Could you check a few things on this model? Use its own coordinates, in mm. A direction names the side the tool comes from. Round coordinates to 2 decimals unless told otherwise and drop trailing zeros. Loops run counter-clockwise (first coordinate to the right, second up) from the corner with the lowest first, then second, coordinate; pieces in that order, holes last. Notation, with made-up numbers: M 3.5,46 L 33.5,46 A19 cw 33.5,79 Z; hole C 22,44.5 d1. An arc over 180 degrees is marked long. One line per item, written item: value. Start each with the question number.
Q1. Imagine slicing it at A-A (y = -36). Please give me the cut outline in (x, z).
Q2. Thinking about a two-plate mould opening in X: for faces 1 (the face through (70, -31, 0)), 2 (the face through (167.5, -49, 1)), 3 (the face through (-13, -100, 52)), which applies, released by +X, released by -X, zero draft, split by the parting line, or undercut?
Q3. Imagine slicing it at B-B (z = 0). Please give me the cut outline in (x, y).
Q4. Which directions (+Z, -Z, +X, -X, +Y, -Y) give clear straight access to the entire face, cutting with the end or side of a thin tool? Please do faces 4 (the face through (2, -30, 21)), 5 (the face through (-167.5, -49, 1)), 6 (the face through (-95, -31, 0)), 7 (the face through (2, -32, -23)).
Q5. Imagine slicing it at C-C (x = 37). Please give me the cut outline in (y, z).
Q6. Please list where these lines run through material, in increasing order: line 1 along Z through (x, y) = (9.5, -41.5); line 2 along X through (y, z) = (-35, 49); line 3 along X through (y, z) = (-18, -37).
Q7. I'm going to push flat-ended pins straight in: pin 1 Ø3 at (x, z) = (66, -17.5) entering from +Y; pin 2 Ø5 at (x, z) = (113, -12) entering from -Y; pin 3 Ø3 at (x, z) = (20.5, -17.5) entering from +Y. Where does each tip first touch, or does it pass through?
Q8. Imagine slicing it at D-D (z = 35). Please give me the cut outline in (x, y), then the cut area to 3 significant figures.
from build123d import *

# Parameters (mm, degrees)
SKETCH2_W           = 335
SKETCH2_H           = 108
BOSS_EXTRUDE4_DEPTH = 100
CUT_EXTRUDE1_DEPTH  = 30
SKETCH4_W           = 300
SKETCH4_H           = 100
CUT_EXTRUDE2_DEPTH  = 68
CUT_EXTRUDE3_DEPTH  = 31


with BuildPart() as part:
    # Sketch2 → Boss-Extrude4 (new body)
    with BuildSketch(Plane(origin=(0, 0, 0), x_dir=(1, 0, 0), z_dir=(0, 1, 0))):
        Rectangle(SKETCH2_W, SKETCH2_H)
    extrude(amount=-BOSS_EXTRUDE4_DEPTH)

    # Sketch3 → Cut-Extrude1 (cut)
    with BuildSketch(Plane(origin=(0, 0, 0), x_dir=(1, 0, 0), z_dir=(0, 1, 0))):
        Polygon((-157.5, -49), (-157.5, 49), (157.5, 39), (157.5, -39), align=None)
    extrude(amount=-CUT_EXTRUDE1_DEPTH, mode=Mode.SUBTRACT)

    # Sketch4 → Cut-Extrude2 (cut)
    with BuildSketch(Plane(origin=(0, -100, 0), x_dir=(-1, 0, 0), z_dir=(0, -1, 0))):
        Rectangle(SKETCH4_W, SKETCH4_H)
    extrude(amount=-CUT_EXTRUDE2_DEPTH, mode=Mode.SUBTRACT)

    # Sketch5 → Cut-Extrude3 (cut)
    with BuildSketch(Plane(origin=(0, -30, 0), x_dir=(1, 0, 0), z_dir=(0, 1, 0))):
        with BuildLine():
            Line((-75, 20), (50, 20))
            ThreePointArc((50, 20), (70, 0), (50, -20))
            Line((50, -20), (-75, -20))
            ThreePointArc((-75, -20), (-95, 0), (-75, 20))
        make_face()
    extrude(amount=-CUT_EXTRUDE3_DEPTH, mode=Mode.SUBTRACT)


solid = part.part
Report:
1. outline: M -167.5,-54 L 167.5,-54 L 167.5,54 L -167.5,54 Z; hole M -150,-50 L 150,-50 L 150,50 L -150,50 Z
2. face 1: undercut
2. face 2: released by +X
2. face 3: zero draft
3. outline: M -167.5,-100 L -150,-100 L -150,-32 L -95,-32 L -95,-30 L -157.5,-30 L -157.5,0 L -167.5,0 Z; M 70,-32 L 150,-32 L 150,-100 L 167.5,-100 L 167.5,0 L 157.5,0 L 157.5,-30 L 70,-30 Z
4. face 4: +Y
4. face 5: +Z, -Z, -X, +Y, -Y
4. face 6: +Y, -Y
4. face 7: -Y
5. outline: M -100,-54 L 0,-54 L 0,-42.83 L -30,-42.83 L -30,-20 L -32,-20 L -32,-50 L -100,-50 Z; M -100,50 L -32,50 L -32,20 L -30,20 L -30,42.83 L 0,42.83 L 0,54 L -100,54 Z
6. line 1: z = -54 to -50, 50 to 54
6. line 2: x = -167.5 to -150, 150 to 167.5
6. line 3: x = -167.5 to -157.5, 157.5 to 167.5
7. pin 1: stops at y = -30
7. pin 2: stops at y = -32
7. pin 3: passes through
8. outline: M -167.5,-100 L -150,-100 L -150,-32 L 150,-32 L 150,-100 L 167.5,-100 L 167.5,0 L 157.5,0 L 157.5,-30 L -157.5,-30 L -157.5,0 L -167.5,0 Z
8. area: 3,650 mm²
